from build123d import *

# Parameters (mm, degrees)
ESQUISSE2_R             = 42.5
ESQUISSE2_R_2           = 39.5
ENL_V_MAT_EXTRU_1_DEPTH = 1.5
ESQUISSE3_R             = 42.5
ESQUISSE3_R_2           = 39.5
ENL_V_MAT_EXTRU_2_DEPTH = 1.5
ENL_V_MAT_EXTRU_3_DEPTH = 4


with BuildPart() as part:
    # Esquisse1 → Révolution1 (revolve)
    with BuildSketch(Plane.XY):
        with BuildLine():
            Line((0, 0), (0, 37.5))
            Line((0, 37.5), (95, 37.5))
            ThreePointArc((95, 37.5), (98.535533906, 38.964466094), (100, 42.5))
            Line((100, 42.5), (200, 42.5))
            ThreePointArc((200, 42.5), (201.464466094, 38.964466094), (205, 37.5))
            Line((205, 37.5), (500, 37.5))
            Line((500, 37.5), (500, 0))
            Line((500, 0), (0, 0))
        make_face()
    revolve(axis=Axis((500, 0, 0), (-1, 0, 0)))

    # Esquisse2 → Enlèv. mat.-Extru.1 (cut)
    with BuildSketch(Plane(origin=(110, 0, 0), x_dir=(0, 0, -1), z_dir=(1, 0, 0))):
        with Locations(Location((0, 0, 0), (0, 0, 90))):
            Circle(ESQUISSE2_R)
        Circle(ESQUISSE2_R_2, mode=Mode.SUBTRACT)
    extrude(amount=-ENL_V_MAT_EXTRU_1_DEPTH, mode=Mode.SUBTRACT)

    # Esquisse3 → Enlèv. mat.-Extru.2 (cut)
    with BuildSketch(Plane(origin=(190, 0, 0), x_dir=(0, 0, -1), z_dir=(1, 0, 0))):
        Circle(ESQUISSE3_R)
        Circle(ESQUISSE3_R_2, mode=Mode.SUBTRACT)
    extrude(amount=-ENL_V_MAT_EXTRU_2_DEPTH, mode=Mode.SUBTRACT)

    # Esquisse4 → Enlèv. mat.-Extru.3 (cut)
    with BuildSketch(Plane(origin=(0, 42.5, 0), x_dir=(1, 0, 0), z_dir=(0, 1, 0))):
        with BuildLine():
            Line((126.75, 8), (171.75, 8))
            ThreePointArc((171.75, 8), (179.75, 0), (171.75, -8))
            Line((171.75, -8), (126.75, -8))
            ThreePointArc((126.75, -8), (118.75, 0), (126.75, 8))
        make_face()
    extrude(amount=-ENL_V_MAT_EXTRU_3_DEPTH, mode=Mode.SUBTRACT)


solid = part.part
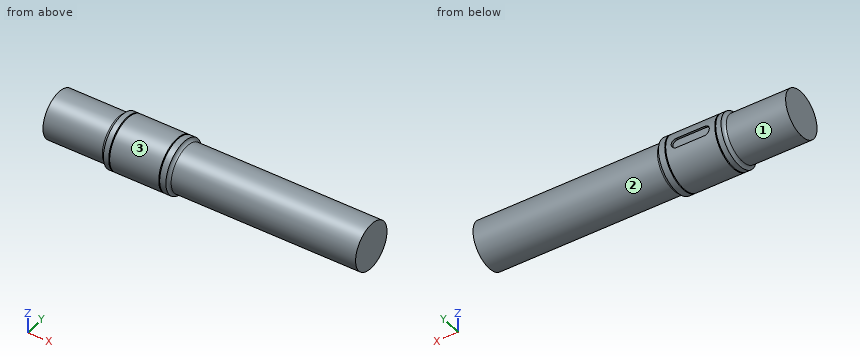
Here's how the part is built. I have some questions about the finished solid (model axes, mm). Face numbers are marked on the shaded views. A direction names the side the tool comes from. Coordinates: 2 decimals unless noted, no trailing zeros. Write each loop counter-clockwise with the first axis right and the second up, starting at its lowest first coordinate (ties: lowest second). Pieces come first, ordered by that corner, then holes.
Item 1: I want a section at B-B on y = 0. Write out the boundary of the cut face in (x, z), and give its area (3 significant figures).
Item 2: I want a section at C-C on x = 422.5. Write out the boundary of the cut face in (y, z), and give its area (3 significant figures).
Item 3: If I drill on line 1 (Y direction, x = 174, z = 0); line 2 (Y direction, x = 261, z = -2); line 3 (Z direction, x = 403.5, y = 29), over which ranges is the centre line in solid material (lowest first)?
Item 4: On a 3-axis mill with a long thin cutter (end or side, diameter ignored), from which of +Z, -Z, +X, -X, +Y, -Y can I reach the whole of each face in a straight line? I mean the marked faces 1, 2 and 3. Say none if no direction works.
Item 5: Will these pins go through, and if not, where does the flat tip stop? pin 1 (1 mm diameter, centred on x = 425, y = 15.5, fed in from +Z); pin 2 (3.5 mm diameter, centred on x = 151, y = 39.5, fed in from +Z); pin 3 (12 mm diameter, centred on x = 190, y = 13.5, fed in from +Z).
Findings below:
1. outline: (0, -37.5) - (95, -37.5) arc R5 cw to (100, -42.5) - (108.5, -42.5) - (108.5, -39.5) - (110, -39.5) - (110, -42.5) - (188.5, -42.5) - (188.5, -39.5) - (190, -39.5) - (190, -42.5) - (200, -42.5) arc R5 cw to (205, -37.5) - (500, -37.5) - (500, 37.5) - (205, 37.5) arc R5 cw to (200, 42.5) - (190, 42.5) - (190, 39.5) - (188.5, 39.5) - (188.5, 42.5) - (110, 42.5) - (110, 39.5) - (108.5, 39.5) - (108.5, 42.5) - (100, 42.5) arc R5 cw to (95, 37.5) - (0, 37.5) - close
1. area: 38,500 mm2
2. outline: circle Ø75 at (0, 0)
2. area: 4,420 mm2
3. line 1: y = -42.5 to 38.5
3. line 2: y = -37.45 to 37.45
3. line 3: z = -23.77 to 23.77
4. face 1: -X
4. face 2: +X
4. face 3: +X, -X
5. pin 1: stops at z = 34.37
5. pin 2: stops at z = 19.52
5. pin 3: stops at z = 41.83
